Could you check a few things on this drawing? It's one solid part, dimensions in mm from its lowest x, y, z. A direction names the side the tool comes from. Coordinates: 2 decimals unless noted, no trailing zeros. Order: outer loops, then holes, each group sorted by start corner. A loop starts at its lowest first (then second) coordinate and runs counter-clockwise, first axis right, second up. Notation, with made-up numbers: M -22,39 L -7,39 A17 cw -7,47 Z; hole C 89,10.25 d4. An arc over 180 degrees is marked long. Answer as CSV lines item,"result". Start each with the question number.
1. If we section it at B-B (z = 5): List the corners of the cut face in (x, y) for me (3 decimals).
2. If we section it at A-A (x = 5): List the corners of the cut face in (y, z) for me (3 decimals), plus the area to 4 significant figures.
3. I need wall thicknesses on line 1 along Z through (x, y) = (5, 2.25); line 2 along Z through (x, y) = (5, 0.8). Which ranges of each line are inside material? Lowest first, please. Write a range as from..to.
4. If we section it at C-C (y = 0.9): List the corners of the cut face in (x, z) for me.
5. On a 3-axis mill with a long thin cutter (end or side, diameter ignored), from which of +Z, -Z, +X, -X, +Y, -Y can I reach the whole of each face in a straight line? I mean the marked faces 1 and 2. Say none if no direction works.
6. If we section it at D-D (y = 2.85): List the corners of the cut face in (x, z) for me, plus the area to 3 significant figures.
7. If we mould it in two halves opening along X, with no side actions, what happens to the marked faces 3, 4, 5 and 6? For each: released by +X, released by -X, zero draft, split by the parting line, or undercut.
8. Will these pins go through, and if not, where does the flat tip stop? pin 1 (2.5 mm diameter, centred on x = 5, z = 3.5, fed in from -Y); pin 2 (2 mm diameter, centred on x = 3, z = 3, fed in from -Y).
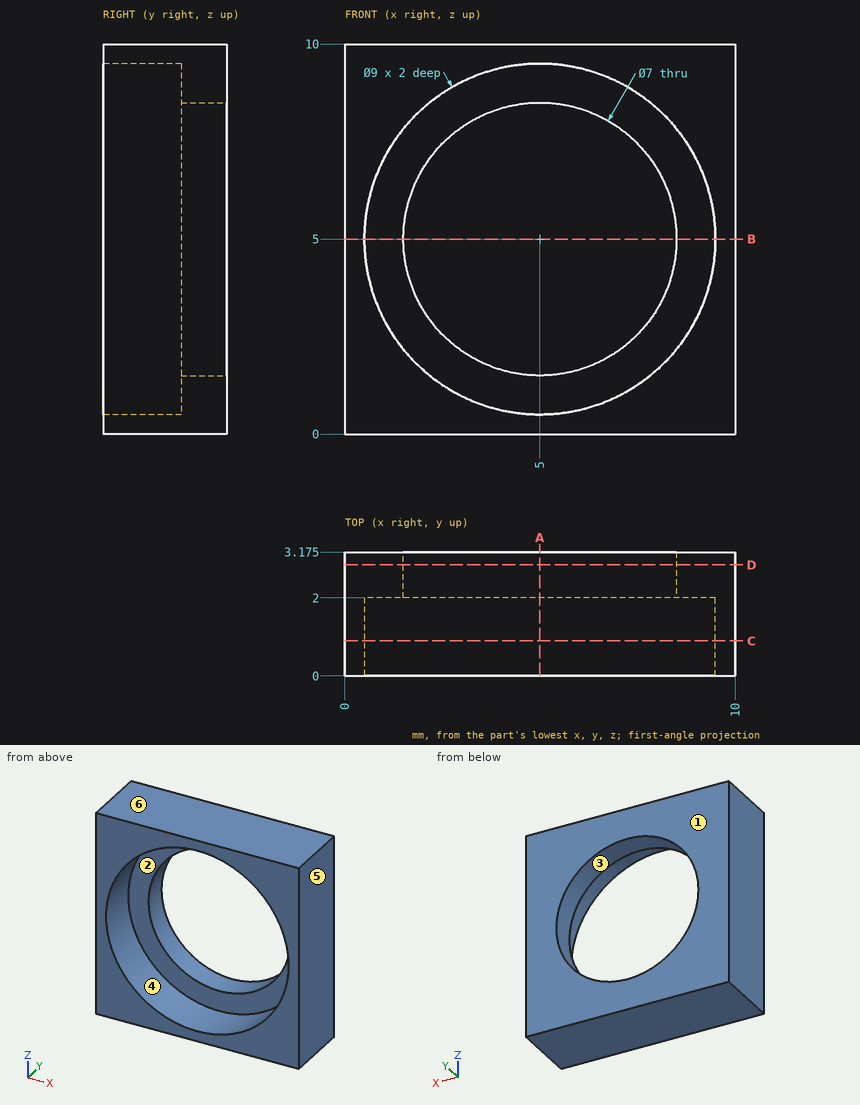
Solved:
1,outline,"M 0,0 L 0.5,0 L 0.5,2 L 1.5,2 L 1.5,3.175 L 0,3.175 Z; M 8.5,2 L 9.5,2 L 9.5,0 L 10,0 L 10,3.175 L 8.5,3.175 Z"
2,outline,"M 0,0 L 3.175,0 L 3.175,1.5 L 2,1.5 L 2,0.5 L 0,0.5 Z; M 0,9.5 L 2,9.5 L 2,8.5 L 3.175,8.5 L 3.175,10 L 0,10 Z"
2,area,"5.525 mm²"
3,line 1,"0..1.5, 8.5..10"
3,line 2,"0..0.5, 9.5..10"
4,outline,"M 0,0 L 10,0 L 10,10 L 0,10 Z; hole C 5,5 d9"
5,face 1,"+Z, -Z, +X, -X, +Y"
5,face 2,"-Y"
6,outline,"M 0,0 L 10,0 L 10,10 L 0,10 Z; hole C 5,5 d7"
6,area,"61.5 mm²"
7,face 3,"undercut"
7,face 4,"undercut"
7,face 5,"released by +X"
7,face 6,"zero draft"
8,pin 1,"through"
8,pin 2,"y = 2"
